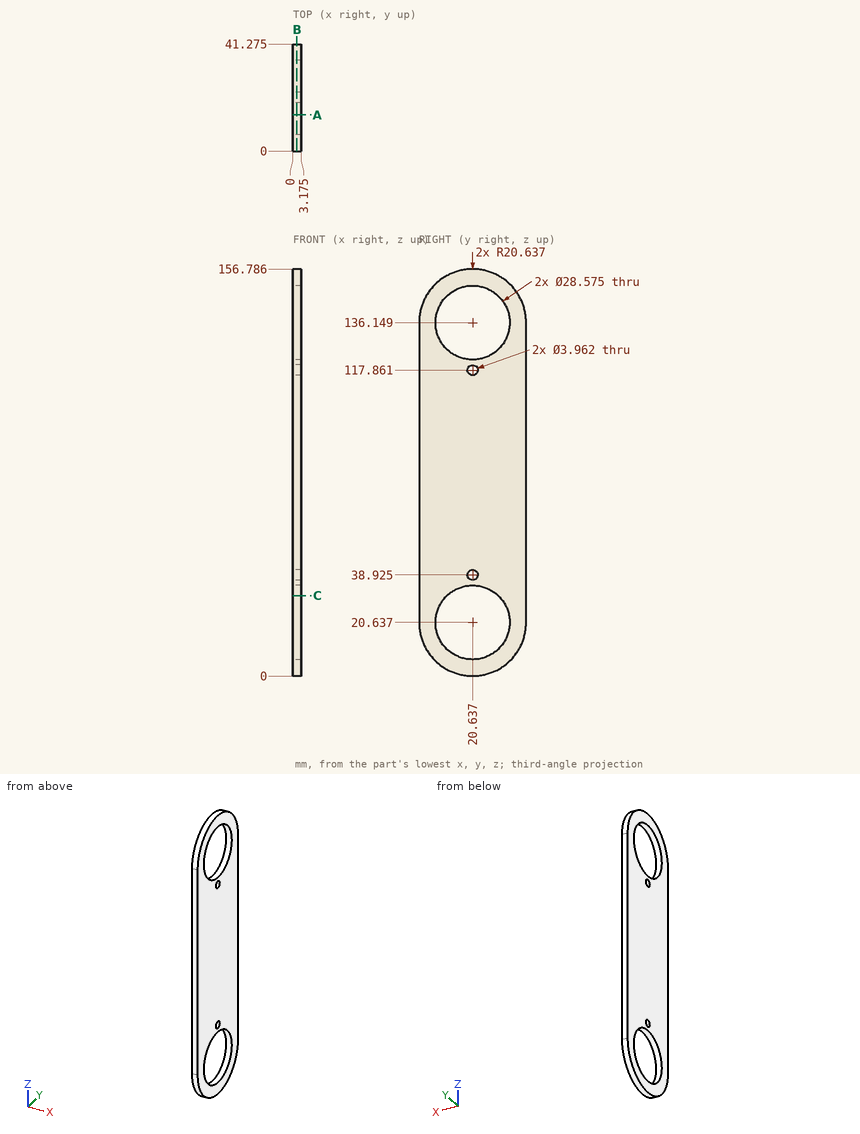
Geometry check sheet. Reference: drawing and pictorial views, mm from the part's lowest x, y, z. Round coordinates to 2 decimals unless told otherwise and drop trailing zeros. Order: outer loops, then holes, each group sorted by start corner. A loop starts at its lowest first (then second) coordinate and runs counter-clockwise, first axis right, second up. Notation, with made-up numbers: M 36,46.25 L 93,46.25 A3 ccw 93,50.25 Z; hole C 60.25,64.25 d5. An arc over 180 degrees is marked long. One line per item, written item: value. Start each with the question number.
1. Gauge pin test, flat ends, axial feed: P1, Ø3, axis at y = 20.64, z = 117.86, coming from the +X side; P2, Ø1.5, axis at x = 1, y = 8, coming from the +Z side. Record the tip position at first contact, or that the pin passes through.
2. Section check B-B on x = 1.55. Give the number of separate pieces and of enclosed holes in the cut face, and give its area (3 significant figures).
3. Scan lines: line 1 along Z through (x, y) = (1.2, 31.5) (1 decimal); line 2 along Z through (x, y) = (1.6, 26) (1 decimal); line 3 along Y through (x, z) = (0.35, 146.5) (1 decimal). Record each from-to range of solid material in increasing order.
4. Section check C-C on z = 31. Enter the section's corners in (x, y) (1 decimal).
5. Section check A-A on y = 14. Enter the section's corners in (x, z) (1 decimal), and give its area (3 significant figures).
Results found:
1. P1: through
1. P2: z = 153.02
2. separate pieces: 1
2. enclosed holes: 4
2. area: 4,800 mm^2
3. line 1: 3.1 to 11.4, 29.9 to 126.9, 145.4 to 153.7
3. line 2: 0.7 to 7.4, 33.9 to 122.9, 149.4 to 156.1
3. line 3: 2.8 to 10.8, 30.5 to 38.5
4. outline: M 0,0 L 3.2,0 L 3.2,10.8 L 0,10.8 Z; M 0,30.5 L 3.2,30.5 L 3.2,41.3 L 0,41.3 Z
5. outline: M 0,1.1 L 3.2,1.1 L 3.2,8 L 0,8 Z; M 0,33.3 L 3.2,33.3 L 3.2,123.5 L 0,123.5 Z; M 0,148.8 L 3.2,148.8 L 3.2,155.7 L 0,155.7 Z
5. area: 330 mm^2
